Part model, mm, in its own coordinate system. Face numbers are marked on the shaded views. A direction names the side the tool comes from. Coordinates: 2 decimals unless noted, no trailing zeros. Write each loop counter-clockwise with the first axis right and the second up, starting at its lowest first coordinate (ties: lowest second). Pieces come first, ordered by that corner, then holes. Notation, with made-up numbers: (73, -13) -> (118, -13) arc R12 cw to (118, -5) -> close; hole circle Ø10 at (18.5, 43). An arc over 180 degrees is marked (long way). One line per question, with ' | ' between items. Start each with the question number.
Item 1: Pin check, flat tips, straight feed: pin 1 (3.5 mm diameter, centred on x = 0.5, z = 13, fed in from +Y); pin 2 (2 mm diameter, centred on x = 23.5, z = 14, fed in from +Y). Stop position of each tip, or through.
Item 2: Saw through at A-A (x = 31.5). List the corners of the cut face in (y, z).
Item 3: Saw through at B-B (z = 20.5). List the corners of the cut face in (x, y), and give its area (3 significant figures).
Item 4: Two-plate mould, pull along Z, no slides. Class the marked faces 1, 2, 3 and 4: pulls with the +Z half, pulls with the -Z half, needs draft (parallel to the pull), parting line crosses it, or undercut.
Item 5: Saw through at D-D (x = 24). List the corners of the cut face in (y, z) (3 decimals).
Item 6: 3-axis set-ups, long thin cutter, end or side, ignore diameter. For the marked faces 5 and 6: which of +Z, -Z, +X, -X, +Y, -Y reach the whole face in a straight line?
Item 7: Probe probe 1 along X at (y, z) = (6.1, 13.5); probe 2 along Z at (x, y) = (24, 2.85) (3 decimals); probe 3 along Z at (x, y) = (0, 6.45). List the from-to ranges inside material, lowest first. Write a range as [from, to].
Item 8: Saw through at C-C (y = 1). Count the separate pieces of the cut face and the enclosed holes in it, and give its area (3 significant figures).
from build123d import *

# Parameters (mm, degrees)
SKETCH1_W           = 52
SKETCH1_H           = 50
SKETCH1_R           = 1.125
SKETCH1_R_2         = 1.65
SKETCH1_W_2         = 40
SKETCH1_H_2         = 21
BOSS_EXTRUDE1_DEPTH = 8
SKETCH2_R           = 2.25
SKETCH2_R_2         = 1.125
CUT_EXTRUDE1_DEPTH  = 3.5


with BuildPart() as part:
    # Sketch1 → Boss-Extrude1 (new body)
    with BuildSketch(Plane(origin=(0, 0, 0), x_dir=(1, 0, 0), z_dir=(0, 1, 0))):
        with Locations((18, 0)):
            Rectangle(SKETCH1_W, SKETCH1_H)
        with Locations((0, 13.5)):
            Circle(SKETCH1_R, mode=Mode.SUBTRACT)
        with Locations((8, 13.5)):
            Circle(SKETCH1_R, mode=Mode.SUBTRACT)
        with Locations((16, 13.5)):
            Circle(SKETCH1_R, mode=Mode.SUBTRACT)
        with Locations((24, 13.5)):
            Circle(SKETCH1_R, mode=Mode.SUBTRACT)
        with Locations((24, -13.5)):
            Circle(SKETCH1_R, mode=Mode.SUBTRACT)
        with Locations((16, -13.5)):
            Circle(SKETCH1_R, mode=Mode.SUBTRACT)
        with Locations((8, -13.5)):
            Circle(SKETCH1_R, mode=Mode.SUBTRACT)
        with Locations((0, -13.5)):
            Circle(SKETCH1_R, mode=Mode.SUBTRACT)
        with Locations((34, 20.5)):
            Circle(SKETCH1_R_2, mode=Mode.SUBTRACT)
        with Locations((2, 20.5)):
            Circle(SKETCH1_R_2, mode=Mode.SUBTRACT)
        with Locations((34, -20.5)):
            Circle(SKETCH1_R_2, mode=Mode.SUBTRACT)
        with Locations((2, -20.5)):
            Circle(SKETCH1_R_2, mode=Mode.SUBTRACT)
        with Locations((18, 0)):
            Rectangle(SKETCH1_W_2, SKETCH1_H_2, mode=Mode.SUBTRACT)
    extrude(amount=BOSS_EXTRUDE1_DEPTH)

    # Sketch2 → Cut-Extrude1 (cut)
    with BuildSketch(Plane(origin=(0, 8, 0), x_dir=(1, 0, 0), z_dir=(0, 1, 0))):
        with Locations((0, 13.5)):
            Circle(SKETCH2_R)
        with Locations((0, 13.5)):
            Circle(SKETCH2_R_2, mode=Mode.SUBTRACT)
        with Locations((8, 13.5)):
            Circle(SKETCH2_R)
        with Locations((8, 13.5)):
            Circle(SKETCH2_R_2, mode=Mode.SUBTRACT)
        with Locations((16, 13.5)):
            Circle(SKETCH2_R)
        with Locations((16, 13.5)):
            Circle(SKETCH2_R_2, mode=Mode.SUBTRACT)
        with Locations((24, 13.5)):
            Circle(SKETCH2_R)
        with Locations((24, 13.5)):
            Circle(SKETCH2_R_2, mode=Mode.SUBTRACT)
        with Locations((24, -13.5)):
            Circle(SKETCH2_R)
        with Locations((24, -13.5)):
            Circle(SKETCH2_R_2, mode=Mode.SUBTRACT)
        with Locations((16, -13.5)):
            Circle(SKETCH2_R)
        with Locations((16, -13.5)):
            Circle(SKETCH2_R_2, mode=Mode.SUBTRACT)
        with Locations((8, -13.5)):
            Circle(SKETCH2_R)
        with Locations((8, -13.5)):
            Circle(SKETCH2_R_2, mode=Mode.SUBTRACT)
        with Locations((0, -13.5)):
            Circle(SKETCH2_R)
        with Locations((0, -13.5)):
            Circle(SKETCH2_R_2, mode=Mode.SUBTRACT)
    extrude(amount=-CUT_EXTRUDE1_DEPTH, mode=Mode.SUBTRACT)


solid = part.part
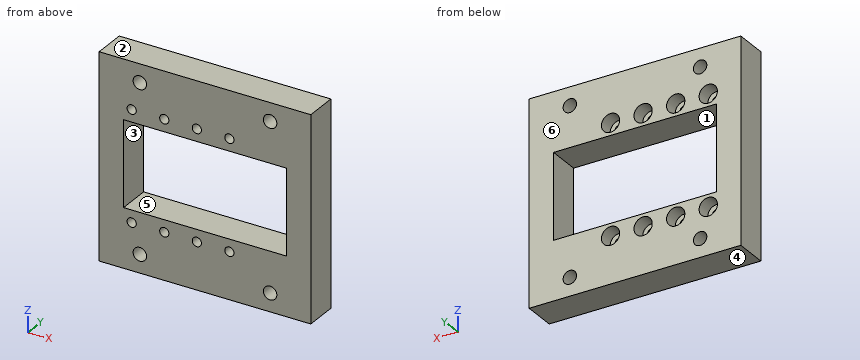
From the geometry:
1) pin 1: y = 8 | pin 2: y = 4.5
2) outline: (0, -25) -> (8, -25) -> (8, -10.5) -> (0, -10.5) -> close; (0, 10.5) -> (8, 10.5) -> (8, 25) -> (0, 25) -> close
3) outline: (-8, 0) -> (0.35, 0) -> (0.35, 8) -> (-8, 8) -> close; (3.65, 0) -> (32.35, 0) -> (32.35, 8) -> (3.65, 8) -> close; (35.65, 0) -> (44, 0) -> (44, 8) -> (35.65, 8) -> close | area: 363 mm2
4) face 1: undercut | face 2: pulls with the +Z half | face 3: undercut | face 4: pulls with the -Z half
5) outline: (0, -25) -> (8, -25) -> (8, -15.75) -> (4.5, -15.75) -> (4.5, -14.625) -> (0, -14.625) -> close; (0, -12.375) -> (4.5, -12.375) -> (4.5, -11.25) -> (8, -11.25) -> (8, -10.5) -> (0, -10.5) -> close; (0, 10.5) -> (8, 10.5) -> (8, 11.25) -> (4.5, 11.25) -> (4.5, 12.375) -> (0, 12.375) -> close; (0, 14.625) -> (4.5, 14.625) -> (4.5, 15.75) -> (8, 15.75) -> (8, 25) -> (0, 25) -> close
6) face 5: +Y, -Y | face 6: +Z, -Z, +X, -X, +Y
7) probe 1: [-8, -2.25], [2.25, 5.75], [10.25, 13.75], [18.25, 21.75], [26.25, 44] | probe 2: [-25, -14.625], [-12.375, -10.5], [10.5, 12.375], [14.625, 25] | probe 3: [-25, -15.75], [-11.25, -10.5], [10.5, 11.25], [15.75, 25]
8) separate pieces: 1 | enclosed holes: 13 | area: 1,690 mm2
